```python
from build123d import *

# Parameters (mm, degrees)
SKETCH1_W           = 76.2
SKETCH1_H           = 70
BOSS_EXTRUDE1_DEPTH = 31
SKETCH2_R           = 6.5
CUT_EXTRUDE1_DEPTH  = 90.400447426
SKETCH4_W           = 56.989038302
SKETCH4_H           = 70
BOSS_EXTRUDE2_DEPTH = 17


with BuildPart() as part:
    # Sketch1 → Boss-Extrude1 (new body)
    with BuildSketch(Plane(origin=(0, 0, 0), x_dir=(1, 0, 0), z_dir=(0, 1, 0))):
        Rectangle(SKETCH1_W, SKETCH1_H)
    extrude(amount=BOSS_EXTRUDE1_DEPTH)

    # Sketch2 → Cut-Extrude1 (cut, through all)
    with BuildSketch(Plane(origin=(38.1, 0, 0), x_dir=(0, 0, -1), z_dir=(1, 0, 0))):
        with Locations((18.1, 15.5)):
            Circle(SKETCH2_R)
    extrude(amount=-CUT_EXTRUDE1_DEPTH, mode=Mode.SUBTRACT)

    # Sketch4 → Boss-Extrude2 (add)
    with BuildSketch(Plane.XZ):
        Rectangle(SKETCH4_W, SKETCH4_H)
    extrude(amount=BOSS_EXTRUDE2_DEPTH)


solid = part.part
```
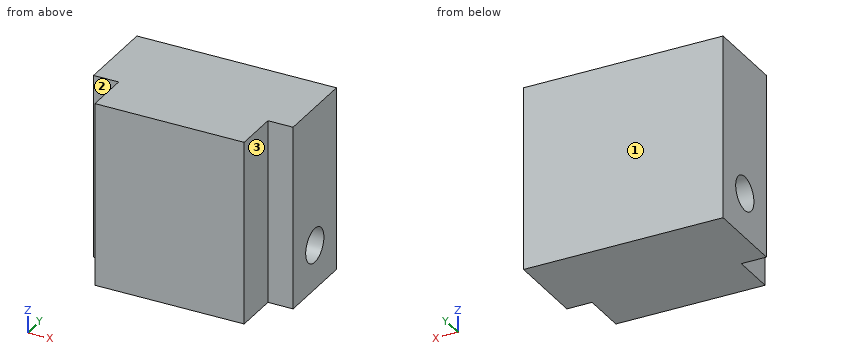
Model file for the job. Use its own axes, mm. Face numbers are marked on the shaded views. A direction names the side the tool comes from. Round coordinates to 2 decimals unless told otherwise and drop trailing zeros. Write each loop counter-clockwise with the first axis right and the second up, starting at its lowest first coordinate (ties: lowest second). Pieces come first, ordered by that corner, then holes. Notation, with made-up numbers: (-15.5, 37) - (15.5, 37) arc R19 cw to (15.5, 70) - close; hole circle Ø8 at (10.25, 37.25). An arc over 180 degrees is marked (long way). Use CSV: the item, a comma, the result in double quotes. Start each with the question number.
Item 1: Band-saw the part on D-D (z = -27.5). Write the cut outline in (x, y).
Item 2: Pin check, flat tips, straight feed: P1, Ø7.5, axis at x = 34, z = -12, coming from the -Y side; P2, Ø18.5, axis at y = -10.5, z = 4, coming from the +X side; P3, Ø13.5, axis at y = -8.5, z = -12, coming from the -X side. Stop position of each tip, or through.
Item 3: Band-saw the part on B-B (y = 15.5). Write the cut outline in (x, z).
Item 4: Band-saw the part on C-C (x = -5.5). Write the cut outline in (y, z), and give its area (3 significant figures).
Item 5: Band-saw the part on A-A (z = -18.1). Write the cut outline in (x, y), and give its area (3 significant figures).
Item 6: Tool access for the marked faces 1, 2 and 3: list every direction of +Z, -Z, +X, -X, +Y, -Y with a clear straight run to the whole face (end or side of a thin tool).
Item 7: Drill centre lines: L1, parallel to Z at x = -32.5, y = 16; L2, parallel to Y at x = -13, z = -18; L3, parallel to Z at x = 20.5, y = 12. Where is each one in solid material? Low to high. Write a range as [from, to].
Checked values:
1,outline,"(-38.1, 0) - (-28.49, 0) - (-28.49, -17) - (28.49, -17) - (28.49, 0) - (38.1, 0) - (38.1, 31) - (-38.1, 31) - close"
2,P1,"stops at y = 0"
2,P2,"stops at x = 28.49"
2,P3,"stops at x = -28.49"
3,outline,"(-38.1, -35) - (38.1, -35) - (38.1, -24.6) - (-38.1, -24.6) - close; (-38.1, -11.6) - (38.1, -11.6) - (38.1, 35) - (-38.1, 35) - close"
4,outline,"(-17, -35) - (31, -35) - (31, 35) - (-17, 35) - close; hole circle Ø13 at (15.5, -18.1)"
4,area,"3,230 mm²"
5,outline,"(-38.1, 0) - (-28.49, 0) - (-28.49, -17) - (28.49, -17) - (28.49, 0) - (38.1, 0) - (38.1, 9) - (-38.1, 9) - close; (-38.1, 22) - (38.1, 22) - (38.1, 31) - (-38.1, 31) - close"
5,area,"2,340 mm²"
6,face 1,"+Z, -Z, +X, -X, +Y"
6,face 2,"+Z, -Z, -X, -Y"
6,face 3,"+Z, -Z, +X, -Y"
7,L1,"z = [-35, -24.58], [-11.62, 35]"
7,L2,"y = [-17, 9], [22, 31]"
7,L3,"z = [-35, -23.58], [-12.62, 35]"
